Build history of the part. All positions in model axes, mm. Coordinates: 2 decimals unless noted, no trailing zeros. Order: outer loops, then holes, each group sorted by start corner. A loop starts at its lowest first (then second) coordinate and runs counter-clockwise, first axis right, second up. Notation, with made-up numbers: (37, -5.5) - (95, -5.5) arc R20 ccw to (95, 13.5) - close; hole circle Ø1 at (8, 76.5). An arc over 180 degrees is marked (long way). Write each question's results on one line, items separated by ' | '.
from build123d import *

# Parameters (mm, degrees)
F0_W     = 419.1
F0_H     = 38.1
F1_DEPTH = 25.4
F3_D     = 15.875
F5_DEPTH = 50.8
F7_DEPTH = 50.8


# Not quite as in the source:
# - a feature names something its author has since deleted; it is built from what else it names


with BuildPart() as f1:
    # F0 (on Front) → F1 (new body)
    with BuildSketch(Plane.XZ):
        with Locations((209.55, 19.05)):
            Rectangle(F0_W, F0_H)
    extrude(amount=F1_DEPTH)

    # F3 (through all)
    with Locations(Plane.XZ.offset(25.4)):
        with Locations((25.4, 19.05), (393.7, 19.05)):
            Hole(F3_D / 2)

    # F4 (on face) → F5 (cut)
    with BuildSketch(Plane.XZ.offset(25.4)):
        Polygon((0, 38.1), (0, 0), (10.2088642316, 38.1), align=None)
    extrude(amount=-F5_DEPTH, mode=Mode.SUBTRACT)

    # F6 (on face) → F7 (cut)
    with BuildSketch(Plane.XZ.offset(25.4)):
        Polygon((419.1, 0), (419.1, 38.1), (408.8911357684, 0), align=None)
    extrude(amount=-F7_DEPTH, mode=Mode.SUBTRACT)


solid = f1.part
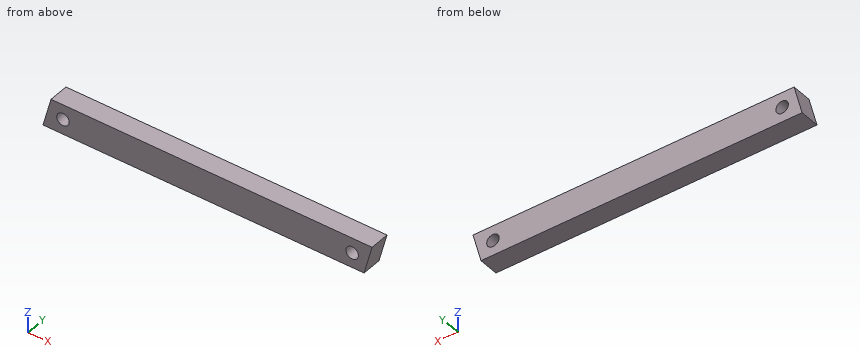
1. Band-saw the part on A-A on x = 393.7. Give the cut face in (y, z), then the cut area to 3 significant figures.
Solved:
outline: (-25.4, 0) - (0, 0) - (0, 11.11) - (-25.4, 11.11) - close; (-25.4, 26.99) - (0, 26.99) - (0, 38.1) - (-25.4, 38.1) - close | area: 565 mm2
2. Band-saw the part on C-C on y = -11.5. Give the number of separate pieces and of enclosed holes in the cut face, then the cut area to 3 significant figures.
Solved:
separate pieces: 1 | enclosed holes: 2 | area: 15,200 mm2
3. Band-saw the part on B-B on z = 19.05. Give the cut face in (x, y).
Solved:
outline: (5.1, -25.4) - (17.46, -25.4) - (17.46, 0) - (5.1, 0) - close; (33.34, -25.4) - (385.76, -25.4) - (385.76, 0) - (33.34, 0) - close; (401.64, -25.4) - (414, -25.4) - (414, 0) - (401.64, 0) - close
4. Drop flat-ended pins along their axis: pin 1 Ø3 at (y, z) = (-12, 23.5) entering from +X; pin 2 Ø12 at (y, z) = (-15, 33) entering from -X. Give the stop position or say it passes through.
Solved:
pin 1: stops at x = 415.59 | pin 2: stops at x = 7.23
5. Probe line 1 (Z direction, x = 25.4, y = -17.5); line 2 (X direction, y = -8.75, z = 17.5); line 3 (X direction, y = -16.75, z = 21). List the from-to ranges inside material, lowest first.
Solved:
line 1: z = 0 to 11.11, 26.99 to 38.1 | line 2: x = 4.69 to 17.62, 33.18 to 385.92, 401.48 to 413.58 | line 3: x = 5.63 to 17.71, 33.09 to 386.01, 401.39 to 414.52
